Build history of the part. All positions in model axes, mm. Give positions to 0.01 mm unless a question says otherwise; leave off trailing zeros. Order: outer loops, then holes, each group sorted by start corner. A loop starts at its lowest first (then second) coordinate and runs counter-clockwise, first axis right, second up. Notation, with made-up numbers: (68, 16.25) - (93, 16.25) arc R16 ccw to (93, 22.25) - close; hole circle Ø10 at (-1.75, 7). An arc over 180 degrees is marked (long way). Use a Markdown table: item, result. Add a question column.
(1) Slice it at C-C (y = 42). Write the cut outline in (x, z), then the cut area to 3 significant figures.
(2) Slice it at A-A (y = 55). Write the cut outline in (x, z) (3 decimals).
(3) Flat gauge pins, fed straight in: pin 1 (2.5 mm diameter, centred on x = 43, y = -34.29, fed in from +Z); pin 2 (2 mm diameter, centred on x = 41.5, z = 0, fed in from +Y); pin 3 (2 mm diameter, centred on x = 47.5, z = -0.5, fed in from +Y). Where does each tip first touch, or does it go through?
(4) Slice it at B-B (x = 7.5). Write the cut outline in (y, z).
(5) Slice it at D-D (x = -9.5). Write the cut outline in (y, z).
(6) Wall check: line 1 (X direction, y = 32, z = 2.5); line 2 (Y direction, x = -23, z = 1.35); line 3 (Y direction, x = -46, z = -0.25). Give the ranges that are in metal, low to high.
from build123d import *

# Parameters (mm, degrees)
SKETCH1_R               = 60
SKETCH1_R_2             = 17.5
BOSS_EXTRUDE2_DEPTH     = 3
FILLET1_R               = 2
CUT_EXTRUDE1_DEPTH      = 86.064681273
CUT_EXTRUDE1_DEPTH_BACK = 86.064681273
CIRPATTERN4_COUNT       = 14


with BuildPart() as part:
    # Sketch1 → Boss-Extrude2 (new, symmetric)
    with BuildSketch(Plane.XY):
        Circle(SKETCH1_R)
        with BuildLine():
            ThreePointArc((-12.023687548, 12.715381935), (-8.75, 15.155444566), (-5, 16.770509831))
            Line((-5, 16.770509831), (-17.5, 46.837484988))
            ThreePointArc((-17.5, 46.837484988), (0, 50), (17.5, 46.837484988))
            Line((17.5, 46.837484988), (5, 16.770509831))
            ThreePointArc((5, 16.770509831), (8.75, 15.155444566), (12.023687548, 12.715381935))
            Line((12.023687548, 12.715381935), (31.812451849, 38.57418706))
            ThreePointArc((31.812451849, 38.57418706), (43.301270189, 25), (49.312451849, 8.263297928))
            Line((49.312451849, 8.263297928), (17.023687548, 4.055127897))
            ThreePointArc((17.023687548, 4.055127897), (17.380513975, 2.041502866), (17.5, 0))
            ThreePointArc((17.5, 0), (17.380513975, -2.041502866), (17.023687548, -4.055127897))
            Line((17.023687548, -4.055127897), (49.312451849, -8.263297928))
            ThreePointArc((49.312451849, -8.263297928), (43.301270189, -25), (31.812451849, -38.57418706))
            Line((31.812451849, -38.57418706), (12.023687548, -12.715381935))
            ThreePointArc((12.023687548, -12.715381935), (8.75, -15.155444566), (5, -16.770509831))
            Line((5, -16.770509831), (17.5, -46.837484988))
            ThreePointArc((17.5, -46.837484988), (0, -50), (-17.5, -46.837484988))
            Line((-17.5, -46.837484988), (-5, -16.770509831))
            ThreePointArc((-5, -16.770509831), (-8.75, -15.155444566), (-12.023687548, -12.715381935))
            Line((-12.023687548, -12.715381935), (-31.812451849, -38.57418706))
            ThreePointArc((-31.812451849, -38.57418706), (-43.301270189, -25), (-49.312451849, -8.263297928))
            Line((-49.312451849, -8.263297928), (-17.023687548, -4.055127897))
            ThreePointArc((-17.023687548, -4.055127897), (-17.5, 0), (-17.023687548, 4.055127897))
            Line((-17.023687548, 4.055127897), (-49.312451849, 8.263297928))
            ThreePointArc((-49.312451849, 8.263297928), (-43.301270189, 25), (-31.812451849, 38.57418706))
            Line((-31.812451849, 38.57418706), (-12.023687548, 12.715381935))
        make_face(mode=Mode.SUBTRACT)
        Circle(SKETCH1_R_2)
    extrude(amount=BOSS_EXTRUDE2_DEPTH, both=True)

    # Fillet1
    fillet1_edges = [part.edges().sort_by_distance(p)[0] for p in [
        (12.023687548, -12.715381935, 0),
        (31.812451849, -38.57418706, 0),
        (49.312451849, -8.263297928, 0),
        (17.023687548, -4.055127897, 0),
        (-17.5, -46.837484988, 0),
        (17.5, -46.837484988, 0),
        (5, -16.770509831, 0),
        (-5, -16.770509831, 0),
        (-49.312451849, -8.263297928, 0),
        (-31.812451849, -38.57418706, 0),
        (-12.023687548, -12.715381935, 0),
        (-17.023687548, -4.055127897, 0),
        (-31.812451849, 38.57418706, 0),
        (-49.312451849, 8.263297928, 0),
        (-17.023687548, 4.055127897, 0),
        (-12.023687548, 12.715381935, 0),
        (17.5, 46.837484988, 0),
        (-17.5, 46.837484988, 0),
        (-5, 16.770509831, 0),
        (5, 16.770509831, 0),
        (49.312451849, 8.263297928, 0),
        (31.812451849, 38.57418706, 0),
        (12.023687548, 12.715381935, 0),
        (17.023687548, 4.055127897, 0),
    ]]
    fillet(fillet1_edges, radius=FILLET1_R)

    # Sketch4 → Cut-Extrude1 (cut, two sides)
    with BuildSketch(Plane(origin=(0, 0, -3), x_dir=(-1, 0, 0), z_dir=(0, 0, -1))) as cut_extrude1_sk:
        with BuildLine():
            Line((-1.1, 1.161895004), (-1.1, -1.161895004))
            ThreePointArc((-1.1, -1.161895004), (1.6, 0), (-1.1, 1.161895004))
        make_face()
    extrude(amount=CUT_EXTRUDE1_DEPTH, mode=Mode.SUBTRACT)
    extrude(cut_extrude1_sk.sketch, amount=-CUT_EXTRUDE1_DEPTH_BACK, mode=Mode.SUBTRACT)

    # Sketch6 → Ø5.0mm Dowel Hole1 (revolve, cut)
    with BuildSketch(Plane(origin=(0, 55, 3), x_dir=(0, -1, 0), z_dir=(1, 0, 0))):
        Polygon((0, 0), (0, 21.016639932), (1.69197298, 20), (1.69197298, 0.83302702), (2.525, 0), align=None)
    f_5_0mm_dowel_hole1 = revolve(axis=Axis((0, 55, 9.35), (0, 0, -1)), mode=Mode.SUBTRACT)

    # CirPattern4: Ø5.0mm Dowel Hole1 ×14 about axis
    cirpattern4_axis = Axis((0, 0, 0), (0, 0, 1))
    for i in range(1, CIRPATTERN4_COUNT):
        add(f_5_0mm_dowel_hole1.rotate(cirpattern4_axis, i * 360 / CIRPATTERN4_COUNT), mode=Mode.SUBTRACT)


solid = part.part
Solution:
| question | item | result |
|---|---|---|
| 1 | outline | (-42.85, -3) - (-15.49, -3) - (-15.49, 3) - (-42.85, 3) - close; (15.49, -3) - (42.85, -3) - (42.85, 3) - (15.49, 3) - close |
| 1 | area | 328 mm2 |
| 2 | outline | (-23.979, -3) - (-1.692, -3) - (-1.692, 2.167) - (-2.525, 3) - (-23.979, 3) - close; (1.692, -3) - (23.979, -3) - (23.979, 3) - (2.525, 3) - (1.692, 2.167) - close |
| 3 | pin 1 | through |
| 3 | pin 2 | y = 44.27 |
| 3 | pin 3 | y = 37.92 |
| 4 | outline | (-59.53, -3) - (-49.43, -3) - (-49.43, 3) - (-59.53, 3) - close; (-22.78, -3) - (22.78, -3) - (22.78, 3) - (-22.78, 3) - close; (49.43, -3) - (59.53, -3) - (59.53, 3) - (49.43, 3) - close |
| 5 | outline | (-59.24, -3) - (-49.09, -3) - (-49.09, 3) - (-59.24, 3) - close; (-27.59, -3) - (27.59, -3) - (27.59, 3) - (-27.59, 3) - close; (49.09, -3) - (59.24, -3) - (59.24, 3) - (49.09, 3) - close |
| 6 | line 1 | -50.75 to -38.42, -26.78 to -11.33, 11.33 to 26.78, 38.42 to 50.75 |
| 6 | line 2 | -55.42 to -51.01, -48.1 to -27.06, -4.83 to 4.83, 27.06 to 48.1, 51.01 to 55.42 |
| 6 | line 3 | -38.52 to -19.6, -7.83 to 7.83, 19.6 to 38.52 |
